Autodesk Inventor part; units mm, degrees
ref_plane "YZ Plane" through (0, 0, 0) normal (1, 0, 0) x (0, 1, 0)
ref_plane "XZ Plane" through (0, 0, 0) normal (0, 1, 0) x (-1, 0, 0)
ref_plane "XY Plane" through (0, 0, 0) normal (0, 0, 1) x (1, 0, 0)
sketch "Sketch1" plane through (0, 0, 0) normal (0, 0, 1) x (1, 0, 0)
  circle A0 centre (0, 0) radius 6.75
  dimension "d0" = 13.5
extrude "Extrusion1" add sketch "Sketch1" along normal blind 15
sketch "Sketch2" plane through (0, 0, 15) normal (0, 0, 1) x (1, 0, 0)
  circle A0 centre (0, 0) radius 11.15
  dimension "d3" = 22.3
extrude "Extrusion3" add sketch "Sketch2" along normal blind 50
sketch "Sketch3" plane through (0, 0, 15) normal (0, 0, -1) x (-1, 0, 0)
  circle A0 centre (0, 0) radius 10.15
  circle A1 centre (0, 0) radius 11.15
  dimension "d8" = 20.3
  dimension "d9" = 22.3
extrude "Extrusion4" add sketch "Sketch3" along normal blind 5
sketch "Sketch4" plane through (0, 0, 65) normal (0, 0, 1) x (1, 0, 0)
  circle A0 centre (0, 0) radius 14.25
  dimension "d12" = 28.5
extrude "Extrusion5" add sketch "Sketch4" along normal blind 20
fillet "Fillet1" radius 2 1 edges at (-14.25, 0, 85)
fillet "Fillet2" radius 2 1 edges at (-6.75, 0, 0)
fillet "Fillet3" radius 2 1 edges at (11.15, 0, 10)
fillet "Fillet4" radius 2 1 edges at (-14.25, 0, 65)
properties part number "Elbow_Parallel_Rod_V1"
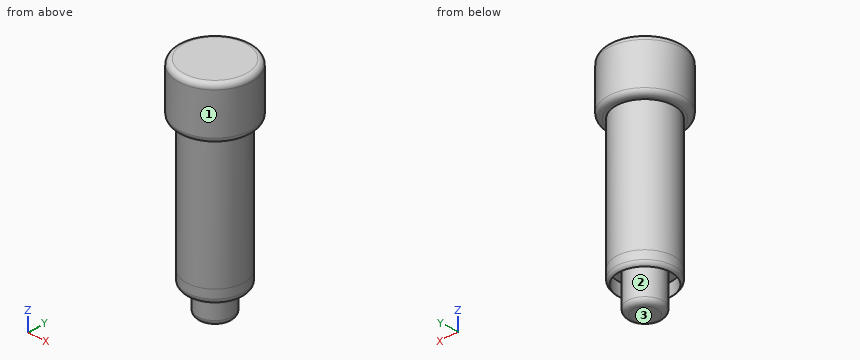
Verification items for the finished model (mm, model axes). Face numbers are marked on the shaded views. Give positions to 0.01 mm unless a question says otherwise; leave off trailing zeros. Loops run counter-clockwise (first coordinate to the right, second up) from the corner with the lowest first, then second, coordinate; pieces in that order, holes last.
1. Section check C-C, the plane z = 74.5. Enter the section's corners in (x, y), then the cut area to 3 significant figures.
2. Thickness scan on line 1 (Y direction, x = 0, z = 11.7); line 2 (X direction, y = 2, z = 14); line 3 (Y direction, x = 1.25, z = 12). Record the ranges inside material, lowest first.
3. Section check D-D, the plane z = 35. Enter the section's corners in (x, y).
4. Section check A-A, the plane x = 0. Enter the section's corners in (y, z), then the cut area to 3 significant figures.
5. Mould release check, pull along Y, two halves, no side actions. Record for the marked faces 1, 2 and 3: released by +Y, released by -Y, zero draft, split by the parting line, or undercut.
6. Go/stop test with flat-tipped pins: pin 1 Ø2 at (x, z) = (-8, 19) entering from +Y; pin 2 Ø12 at (y, z) = (6.5, 19) entering from +X; pin 3 Ø2 at (x, y) = (11.5, -6) entering from +Z; pin 4 Ø12 at (y, z) = (2, 26.5) entering from -X. Record where each tip stops, or that it passes through.
Geometry says:
1. outline: circle Ø28.5 at (0, 0)
1. area: 638 mm2
2. line 1: y = -11.15 to -10.15, -6.75 to 6.75, 10.15 to 11.15
2. line 2: x = -10.97 to -9.95, -6.45 to 6.45, 9.95 to 10.97
2. line 3: y = -11.08 to -10.07, -6.63 to 6.63, 10.07 to 11.08
3. outline: circle Ø22.3 at (0, 0)
4. outline: (-14.25, 67) arc R2 ccw to (-12.25, 65) - (-11.15, 65) - (-11.15, 11.73) arc R2 ccw to (-10.15, 10) - (-10.15, 15) - (-6.75, 15) - (-6.75, 2) arc R2 ccw to (-4.75, 0) - (4.75, 0) arc R2 ccw to (6.75, 2) - (6.75, 15) - (10.15, 15) - (10.15, 10) arc R2 ccw to (11.15, 11.73) - (11.15, 65) - (12.25, 65) arc R2 ccw to (14.25, 67) - (14.25, 83) arc R2 ccw to (12.25, 85) - (-12.25, 85) arc R2 ccw to (-14.25, 83) - close
4. area: 1,890 mm2
5. face 1: split by the parting line
5. face 2: undercut
5. face 3: zero draft
6. pin 1: stops at y = 8.68
6. pin 2: stops at x = 11.14
6. pin 3: stops at z = 85
6. pin 4: stops at x = -11.15
